Geometry: see drawing. Coordinates: mm, zero at the bounding-box minimum. Give positions to 0.01 mm unless a question says otherwise; leave off trailing zeros. Write each loop counter-clockwise with the first axis right and the second up, starting at its lowest first coordinate (ties: lowest second). Pieces come first, ordered by that corner, then holes. Notation, with made-up numbers: (29, 36.25) - (45, 36.25) arc R8 cw to (45, 40.25) - close; hole circle Ø8 at (86, 53.25). An arc over 180 degrees is marked (long way). Use CSV: the item, a comma, the result in double quotes. Start each with the question number.
(1) Section C-C on x = 75. Output: boundary loops of the cut face in (y, z).
(2) Section B-B on y = 1.35. Output: boundary loops of the cut face in (x, z), and give its area (3 significant figures).
(3) First-contact query: pin 1 Ø3 at (x, y) = (102, 2) entering from -Z; pin 2 Ø1.5 at (x, y) = (90, 4.5) entering from +Z; pin 3 Ø3 at (x, y) = (22.5, 4) entering from +Z. Flat tips, straight axial feed; report the tip coordinate or a pass-through.
(4) Section A-A on z = 75. Output: boundary loops of the cut face in (x, y).
(5) Line query: probe 1 along X at (y, z) = (0.8, 115); probe 2 along X at (y, z) = (4.3, 68.5); probe 3 along Z at (x, y) = (70.5, 1.65). Output: solid intervals per line, ascending. Write a range as [from, to].
(6) Section D-D on z = 115. Output: boundary loops of the cut face in (x, y).
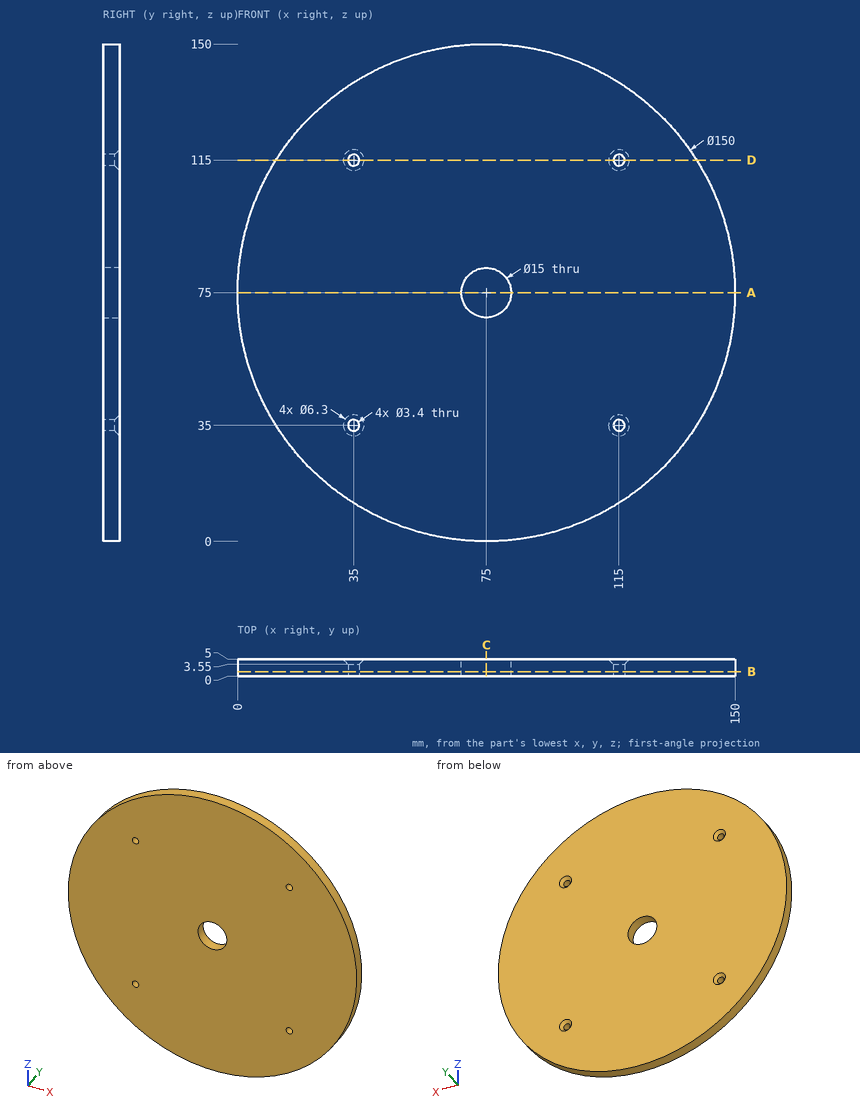
Check values:
1,outline,"(0, 0) - (5, 0) - (5, 67.5) - (0, 67.5) - close; (0, 82.5) - (5, 82.5) - (5, 150) - (0, 150) - close"
2,outline,"circle Ø150 at (75, 75); hole circle Ø3.4 at (35, 35); hole circle Ø3.4 at (35, 115); hole circle Ø15 at (75, 75); hole circle Ø3.4 at (115, 35); hole circle Ø3.4 at (115, 115)"
2,area,"17,500 mm²"
3,pin 1,"stops at z = 4.47"
3,pin 2,"stops at z = 148.63"
3,pin 3,"stops at z = 129.99"
4,outline,"(0, 0) - (67.5, 0) - (67.5, 5) - (0, 5) - close; (82.5, 0) - (150, 0) - (150, 5) - (82.5, 5) - close"
5,probe 1,"x = [11.56, 33.3], [36.7, 113.3], [116.7, 138.44]"
5,probe 2,"x = [0.28, 71.26], [78.74, 149.72]"
5,probe 3,"z = [0.14, 69], [81, 149.86]"
6,outline,"(11.56, 0) - (33.3, 0) - (33.3, 3.55) - (31.85, 5) - (11.56, 5) - close; (36.7, 0) - (113.3, 0) - (113.3, 3.55) - (111.85, 5) - (38.15, 5) - (36.7, 3.55) - close; (116.7, 0) - (138.44, 0) - (138.44, 5) - (118.15, 5) - (116.7, 3.55) - close"
